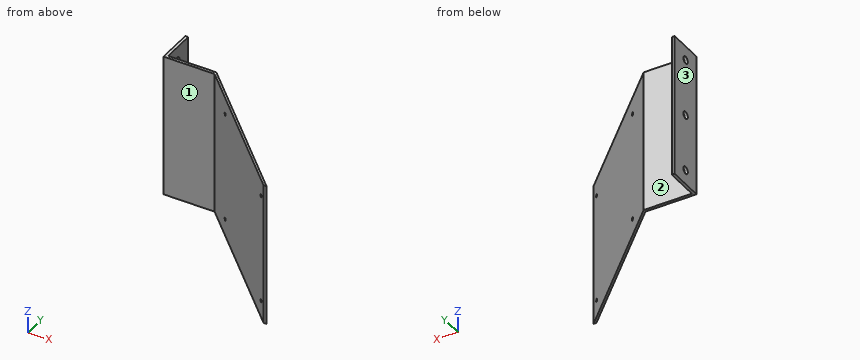
```python
from build123d import *

# Parameters (mm, degrees)
SKETCH1_W               = 33.68957
SKETCH1_H               = 2.032
SKETCH1_W_2             = 2.032
SKETCH1_H_2             = 23.368
BOSS_EXTRUDE1_DEPTH     = 100
CUT_EXTRUDE1_DEPTH      = 159.384645446
CUT_EXTRUDE1_DEPTH_BACK = 159.384645446
SKETCH2_R               = 1.13
F_4_40_TAPPED_HOLE1_D   = 2.2606
F_1_4_20_TAPPED_HOLE1_D = 5.1054


with BuildPart() as part:
    # Sketch1 → Boss-Extrude1 (new body)
    with BuildSketch(Plane.XY):
        Polygon((0, 2.032), (0, 0), (85.833570848, -85.833570848), (87.865570848, -85.833570848), align=None)
        with Locations((-16.844785, 1.016)):
            Rectangle(SKETCH1_W, SKETCH1_H)
        with Locations((-34.70557, 13.716)):
            Rectangle(SKETCH1_W_2, SKETCH1_H_2)
        with Locations((-34.70557, 1.016)):
            Rectangle(SKETCH1_W_2, SKETCH1_H)
        Polygon((85.833570848, -85.833570848), (87.865570848, -85.833570848), (0, 2.032), (0, 0), align=None)
    extrude(amount=BOSS_EXTRUDE1_DEPTH)

    # Sketch2 → Cut-Extrude1 (cut, two sides: drawn at the far end of the back side and taken through both)
    with BuildSketch(Plane(origin=(1.016, 1.016, 0), x_dir=(0, 0, -1), z_dir=(0.707106781186546, 0.707106781186549, 0)).offset(-CUT_EXTRUDE1_DEPTH_BACK)):
        with Locations(Location((-88.1, -26.137000979, 0), (0, 0, 90))):
            Circle(SKETCH2_R)
        with Locations(Location((-11.9, -26.137000979, 0), (0, 0, 90))):
            Circle(SKETCH2_R)
        with Locations(Location((-11.9, -115.037000979, 0), (0, 0, 90))):
            Circle(SKETCH2_R)
        with Locations(Location((-88.1, -115.037000979, 0), (0, 0, 90))):
            Circle(SKETCH2_R)
    extrude(amount=CUT_EXTRUDE1_DEPTH + CUT_EXTRUDE1_DEPTH_BACK, mode=Mode.SUBTRACT)

    # 4-40 Tapped Hole1 (through all)
    with Locations(Plane(origin=(19.497650632, -17.465650632, 88.1), x_dir=(0.707106781187, -0.707106781187, 0), z_dir=(0.707106781187, 0.707106781187, 0))):
        with Locations((1e-09, 0), (1e-09, 76.2), (88.900000001, 76.2), (88.900000001, 0)):
            Hole(F_4_40_TAPPED_HOLE1_D / 2)

    # 1_4-20 Tapped Hole1 (through all)
    with Locations(Plane.ZY.offset(35.72157)):
        with Locations((10, 12.7), (50, 12.7), (90, 12.7)):
            Hole(F_1_4_20_TAPPED_HOLE1_D / 2)


solid = part.part
```
Input: part model. Units: mm. Frame: model coordinates. Face numbers are marked on the shaded views. A direction names the side the tool comes from. Coordinates: 2 decimals unless noted, no trailing zeros. Write each loop counter-clockwise with the first axis right and the second up, starting at its lowest first coordinate (ties: lowest second). Pieces come first, ordered by that corner, then holes.
1) Section C-C on z = 73.5. Output: boundary loops of the cut face in (x, y), and give its area (3 significant figures).
2) Material intervals for line 1 along Y through (x, z) = (-34, 90); line 2 along X through (y, z) = (19, 18.5); line 3 along Y through (x, z) = (-21.5, 70.5), sorted ascending.
3) Section B-B on y = 12.7. Output: boundary loops of the cut face in (x, z), and give its area (3 significant figures).
4) Set-up query: the marked faces 1, 2 and 3. Return all of +Z, -Z, +X, -X, +Y, -Y with unobstructed straight access to the full face (end or side cutting, diameter ignored); none if empty.
5) Pin query (flat end, axial travel): pin 1 Ø12 at (x, z) = (21.5, 75) entering from +Y; pin 2 Ø10 at (x, z) = (-20.5, 60) entering from +Y; pin 3 Ø1.5 at (y, z) = (-40, 79) entering from -X; pin 4 Ø8 at (y, z) = (12.7, 90) entering from -X. Return the tip coordinate at first contact, or that it passes through.
6) Section A-A on z = 50. Output: boundary loops of the cut face in (x, y).
7) Section D-D on x = 26.5. Output: boundary loops of the cut face in (y, z).
Check result:
1. outline: (-35.72, 0) - (0, 0) - (85.83, -85.83) - (87.87, -85.83) - (0, 2.03) - (-33.69, 2.03) - (-33.69, 25.4) - (-35.72, 25.4) - close
1. area: 297 mm2
2. line 1: y = 0 to 10.15, 15.25 to 25.4
2. line 2: x = -35.72 to -33.69
2. line 3: y = 0 to 2.03
3. outline: (-35.72, 0) - (-33.69, 0) - (-33.69, 7.45) - (-35.72, 7.45) - close; (-35.72, 12.55) - (-33.69, 12.55) - (-33.69, 47.45) - (-35.72, 47.45) - close; (-35.72, 52.55) - (-33.69, 52.55) - (-33.69, 87.45) - (-35.72, 87.45) - close; (-35.72, 92.55) - (-33.69, 92.55) - (-33.69, 100) - (-35.72, 100) - close
3. area: 172 mm2
4. face 1: +Z, -Z, -X, -Y
4. face 2: +Z, -Z, +X, +Y
4. face 3: +Z, -Z, -X, +Y, -Y
5. pin 1: stops at y = -13.47
5. pin 2: stops at y = 2.03
5. pin 3: stops at x = 39.25
5. pin 4: stops at x = -35.72
6. outline: (-35.72, 0) - (0, 0) - (85.83, -85.83) - (87.87, -85.83) - (0, 2.03) - (-33.69, 2.03) - (-33.69, 10.15) - (-35.72, 10.15) - close; (-35.72, 15.25) - (-33.69, 15.25) - (-33.69, 25.4) - (-35.72, 25.4) - close
7. outline: (-26.5, 0) - (-24.47, 0) - (-24.47, 100) - (-26.5, 100) - close
